Could you check a few things on this model? Use its own coordinates, in mm. Face numbers are marked on the shaded views. A direction names the side the tool comes from. Give positions to 0.01 mm unless a question says otherwise; leave off trailing zeros. Loops run counter-clockwise (first coordinate to the right, second up) from the corner with the lowest first, then second, coordinate; pieces in that order, holes last. Notation, with made-up numbers: (41, 11.25) - (50, 11.25) arc R15 cw to (50, 22.25) - close; hole circle Ø2 at (-20, -39.75). An arc over 180 degrees is marked (long way). Use CSV: the item, a comma, the result in double quotes.
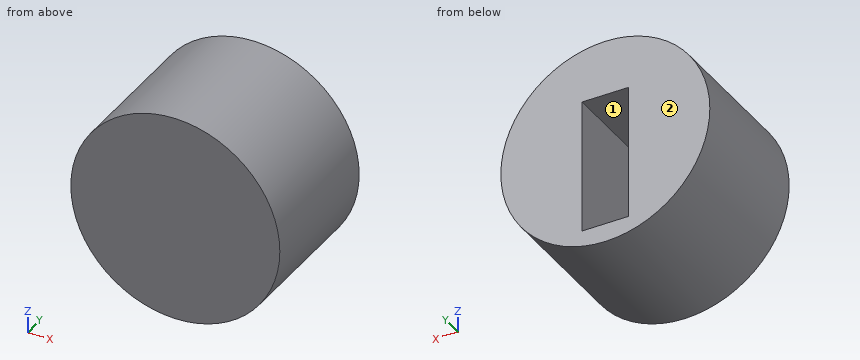
from build123d import *

# Parameters (mm, degrees)
SKETCH1_R           = 45
BOSS_EXTRUDE1_DEPTH = 60
SKETCH2_W           = 20
SKETCH2_H           = 58
CUT_EXTRUDE1_DEPTH  = 40


with BuildPart() as part:
    # Sketch1 → Boss-Extrude1 (new body)
    with BuildSketch(Plane(origin=(0, 0, 0), x_dir=(1, 0, 0), z_dir=(0, 1, 0))):
        with Locations(Location((0, 0, 0), (0, 0, 270))):
            Circle(SKETCH1_R)
    extrude(amount=BOSS_EXTRUDE1_DEPTH)

    # Sketch2 → Cut-Extrude1 (cut)
    with BuildSketch(Plane(origin=(0, 60, 0), x_dir=(1, 0, 0), z_dir=(0, 1, 0))):
        with Locations((0, 8)):
            Rectangle(SKETCH2_W, SKETCH2_H)
    extrude(amount=-CUT_EXTRUDE1_DEPTH, mode=Mode.SUBTRACT)


solid = part.part
1) Suppose I cut it at A-A (z = 0). Please give me the cut outline in (x, y).
Answer below:
outline,"(-45, 0) - (45, 0) - (45, 60) - (10, 60) - (10, 20) - (-10, 20) - (-10, 60) - (-45, 60) - close"
2) Which directions (+Z, -Z, +X, -X, +Y, -Y) give clear straight access to the entire face, cutting with the end or side of a thin tool? Please do the marked faces 1 and 2.
Answer below:
face 1,"+Y"
face 2,"+Z, -Z, +X, -X, +Y"
3) I'm going to push flat-ended pins straight in: P1, Ø8, axis at x = -13, y = 31, coming from the -Z side; P2, Ø4, axis at y = 20.5, z = 18, coming from the -X side; P3, Ø5, axis at x = 1, y = 45.5, coming from the +Z side; P4, Ø1, axis at y = 45.5, z = -2.5, coming from the +X side. Where does each tip first touch, or does it pass through?
Answer below:
P1,"stops at z = -44.09"
P2,"stops at x = -42.06"
P3,"stops at z = 45"
P4,"stops at x = 44.96"
4) I need wall thicknesses on line 1 along Y through (x, z) = (-5.5, 17.5); line 2 along X through (y, z) = (29, 16); line 3 along Z through (x, y) = (1.5, 35) (3 decimals). Which ranges of each line are inside material? Lowest first, please.
Answer below:
line 1,"y = 0 to 20"
line 2,"x = -42.06 to -10, 10 to 42.06"
line 3,"z = -44.975 to -37, 21 to 44.975"
5) Suppose I cut it at D-D (y = 12). Please give me the cut outline in (x, z), plus the area to 3 significant figures.
Answer below:
outline,"circle Ø90 at (0, 0)"
area,"6,360 mm2"
6) Suppose I cut it at B-B (y = 48.5). Please give me the cut outline in (x, z).
Answer below:
outline,"circle Ø90 at (0, 0); hole (-10, -37) - (10, -37) - (10, 21) - (-10, 21) - close"
7) Suppose I cut it at C-C (x = 0). Please give me the cut outline in (y, z).
Answer below:
outline,"(0, -45) - (60, -45) - (60, -37) - (20, -37) - (20, 21) - (60, 21) - (60, 45) - (0, 45) - close"
